```python
from build123d import *

# Parameters (mm, degrees)
BOX002_W         = 6
BOX002_H         = 10
BOX002_DEPTH     = 13
ARRAY003_X_COUNT = 2
ARRAY003_X_PITCH = 506
ARRAY003_Z_COUNT = 2
ARRAY003_Z_PITCH = 26
BOX001_W         = 26.3157894737
BOX001_H         = 10
BOX001_DEPTH     = 6
ARRAY001_X_COUNT = 10
ARRAY001_X_PITCH = 52.6315789474
BOX_W            = 512
BOX_H            = 6
BOX_DEPTH        = 39


with BuildPart() as vertical_array:
    # Box002 → Box002 (new body)
    with BuildSketch(Plane.XY):
        with Locations((3, 5)):
            Rectangle(BOX002_W, BOX002_H)
    extrude(amount=BOX002_DEPTH)

    # Array003 X: Vertical_Array ×2


with BuildPart() as vertical_array_1:
    add(vertical_array.part)
    with Locations(*[(i * ARRAY003_X_PITCH, 0, 0) for i in range(1, ARRAY003_X_COUNT)]):
        add(vertical_array.part)

    # Array003 Z: Vertical_Array ×2


with BuildPart() as vertical_array_2:
    add(vertical_array_1.part)
    with Locations(*[(0, 0, i * ARRAY003_Z_PITCH) for i in range(1, ARRAY003_Z_COUNT)]):
        add(vertical_array_1.part)


with BuildPart() as horizontal_array:
    # Box001 → Box001 (new body)
    with BuildSketch(Plane.XY):
        with Locations((13.1578947368, 5)):
            Rectangle(BOX001_W, BOX001_H)
    extrude(amount=BOX001_DEPTH)

    # Array001 X: Horizontal_Array ×10


with BuildPart() as horizontal_array_1:
    add(horizontal_array.part)
    with Locations(*[(i * ARRAY001_X_PITCH, 0, 0) for i in range(1, ARRAY001_X_COUNT)]):
        add(horizontal_array.part)


with BuildPart() as horizontal_array_2:
    # Array001 placement: moved
    add(horizontal_array_1.part.moved(Location((6, 0, 0))))


with BuildPart() as cut001:
    # Box → Box (new body)
    with BuildSketch(Plane.XY):
        with Locations((256, 3)):
            Rectangle(BOX_W, BOX_H)
    extrude(amount=BOX_DEPTH)

    # Cut: cut Horizontal_Array
    add(horizontal_array_2.part, mode=Mode.SUBTRACT)

    # Cut001: cut Vertical_Array
    add(vertical_array_2.part, mode=Mode.SUBTRACT)


solid = cut001.part
```
Input: part model. Units: mm. Frame: model coordinates. Give positions to 0.01 mm unless a question says otherwise; leave off trailing zeros. Loops run counter-clockwise (first coordinate to the right, second up) from the corner with the lowest first, then second, coordinate; pieces in that order, holes last.
1) Contact query for flat-ended pins moving along their axis: pin 1 (1.8 mm diameter, centred on y = 2.5, z = 4, fed in from +X); pin 2 (3 mm diameter, centred on x = 509.5, y = 3.5, fed in from -Z); pin 3 (1.5 mm diameter, centred on x = 280, y = 1.5, fed in from -Z). Output: stop coordinate, or through.
A:
pin 1: stops at x = 479.68
pin 2: stops at z = 13
pin 3: stops at z = 6
2) Line query: L1, parallel to X at y = 4, z = 28; L2, parallel to Z at x = 164, y = 2.4. Output: solid intervals per line, ascending.
A:
L1: x = 6 to 506
L2: z = 6 to 39
3) Section query A-A on x = 435. Return the cut outline in (y, z), and give its area (3 significant figures).
A:
outline: (0, 6) - (6, 6) - (6, 39) - (0, 39) - close
area: 198 mm2
